The model under review builds one solid part; all positions refer to its coordinate system, in mm. A direction names the side the tool comes from. Round coordinates to 2 decimals unless told otherwise and drop trailing zeros. Loops run counter-clockwise (first coordinate to the right, second up) from the corner with the lowest first, then second, coordinate; pieces in that order, holes last. Notation, with made-up numbers: M 74.5,88.5 L 104.5,88.5 A20 ccw 104.5,96.5 Z; hole C 28,53 d3. An arc over 180 degrees is marked long. Return JSON: item names as keys, results as strings. Group by question number.
Q1. Consider section B-B (x = -6). State the section outline as (y, z) points.
Q2. Consider section A-A (z = -6). State the section outline as (x, y) points.
Q3. Consider section D-D (z = 10.5). State the section outline as (x, y) points, and give its area (3 significant figures).
Q4. To check wall thickness, follow line 1 along X through (y, z) = (1.5, -6); line 2 along X through (y, z) = (3.25, -15); line 3 along Z through (x, y) = (5, 1). State the ranges of each line that lie inside material, in increasing order.
Q5. Clearance check with flat-ended pins moving along their axes: pin 1 Ø1.8 at (y, z) = (3.5, 14.5) entering from +X; pin 2 Ø5.5 at (x, z) = (4, -6) entering from -Y; pin 3 Ø1 at (y, z) = (3.5, 3.5) entering from -X; pin 4 Ø5.5 at (x, z) = (-8, -7) entering from -Y. State where each tip first meets the part, or that it passes through.
Q6. Consider section C-C (y = 5). State the section outline as (x, z) points (3 decimals).
Q7. Draft analysis for pull direction Z (two halves, no side actions). For faces 5 (the face through (21, 3, 5)), 6 (the face through (4, 4, -4)), 7 (the face through (-9, 5, -21)), 8 (the face through (-13.12, 0.64, -18.03)), state which applies: pulls with the +Z half, pulls with the -Z half, needs draft (parallel to the pull), parting line crosses it, or undercut.
Q8. For faces 1 (the face through (-18, 1.3, -10)), 2 (the face through (-8.48, 4.99, 8.12)), 3 (the face through (6.828, 3, 14)), 4 (the face through (-3.97, 5.01, 1.79)), list the 3-axis set-ups (+Z, -Z, +X, -X, +Y, -Y) from which the entire face can be reached by the end or side of a thin tool; tool diameter is ignored.
from build123d import *

# Parameters (mm, degrees)
SKETCH2_W           = 44
SKETCH2_H           = 44
BOSS_EXTRUDE1_DEPTH = 6
CHAMFER1_SIZE       = 18
SKETCH3_R           = 8
CUT_EXTRUDE1_DEPTH  = 32.685959036
SKETCH4_R           = 9.1
CUT_EXTRUDE2_DEPTH  = 1.3
CUT_EXTRUDE3_DEPTH  = 32.685959036
SKETCH7_R           = 1.7
CUT_EXTRUDE4_DEPTH  = 32.685959036
SKETCH8_R           = 3
CUT_EXTRUDE5_DEPTH  = 2
CHAMFER2_SIZE       = 2


with BuildPart() as part:
    # Sketch2 → Boss-Extrude1 (new body)
    with BuildSketch(Plane(origin=(0, 0, 0), x_dir=(1, 0, 0), z_dir=(0, 1, 0))):
        Rectangle(SKETCH2_W, SKETCH2_H)
    extrude(amount=BOSS_EXTRUDE1_DEPTH)

    # Chamfer1
    chamfer1_edges = [part.edges().sort_by_distance(p)[0] for p in [
        (22, 3, 22),
    ]]
    chamfer(chamfer1_edges, length=CHAMFER1_SIZE)

    # Sketch3 → Cut-Extrude1 (cut, through all)
    with BuildSketch(Plane(origin=(0, 6, 0), x_dir=(1, 0, 0), z_dir=(0, 1, 0))):
        with Locations(Location((-9.629833996, 9.625, 0), (0, 0, 270))):
            Circle(SKETCH3_R)
    extrude(amount=-CUT_EXTRUDE1_DEPTH, mode=Mode.SUBTRACT)

    # Sketch4 → Cut-Extrude2 (cut)
    with BuildSketch(Plane(origin=(0, 0, 0), x_dir=(-1, 0, 0), z_dir=(0, -1, 0))):
        with Locations(Location((9.629833996, 9.625, 0), (0, 0, 90))):
            Circle(SKETCH4_R)
    extrude(amount=-CUT_EXTRUDE2_DEPTH, mode=Mode.SUBTRACT)

    # Sketch5 → Cut-Extrude3 (cut, through all)
    with BuildSketch(Plane(origin=(0, 6, 0), x_dir=(1, 0, 0), z_dir=(0, 1, 0))):
        Polygon((-14, 22), (-22, 14), (-22, 22), align=None)
    extrude(amount=-CUT_EXTRUDE3_DEPTH, mode=Mode.SUBTRACT)

    # Sketch7 → Cut-Extrude4 (cut, through all)
    with BuildSketch(Plane(origin=(0, 6, 0), x_dir=(1, 0, 0), z_dir=(0, 1, 0))):
        with Locations(Location((4, 6, 0), (0, 0, 270))):
            Circle(SKETCH7_R)
        with Locations(Location((-6, -4, 0), (0, 0, 270))):
            Circle(SKETCH7_R)
        Polygon((-4, 22), (22, -4), (22, 22), align=None)
        Polygon((-22, 4), (4, -22), (-22, -22), align=None)
        Polygon((19.171572875, -6.828427125), (9.656854249, -6.828427125), (6.828427125, -9.656854249), (6.828427125, -19.171572875), align=None)
    extrude(amount=-CUT_EXTRUDE4_DEPTH, mode=Mode.SUBTRACT)

    # Sketch8 → Cut-Extrude5 (cut)
    with BuildSketch(Plane(origin=(0, 6, 0), x_dir=(1, 0, 0), z_dir=(0, 1, 0))):
        with Locations(Location((4, 6, 0), (0, 0, 270))):
            Circle(SKETCH8_R)
        with Locations(Location((-6, -4, 0), (0, 0, 270))):
            Circle(SKETCH8_R)
    extrude(amount=-CUT_EXTRUDE5_DEPTH, mode=Mode.SUBTRACT)

    # Chamfer2
    chamfer2_edges = [part.edges().sort_by_distance(p)[0] for p in [
        (-22, 6, -9),
        (-18, 6, -18),
        (-9, 6, -22),
        (-9, 6, 9),
        (9, 6, -9),
    ]]
    chamfer(chamfer2_edges, length=CHAMFER2_SIZE)


solid = part.part
Values:
{
 "1": {"outline": "M 0,-22 L 4,-22 L 6,-20 L 6,-16.75 L 1.3,-16.75 L 1.3,-17.97 L 0,-17.97 Z; M 0,-1.28 L 1.3,-1.28 L 1.3,-2.5 L 6,-2.5 L 6,1 L 4,1 L 4,2.3 L 0,2.3 Z; M 0,5.7 L 4,5.7 L 4,7 L 6,7 L 6,9.17 L 4,12 L 0,12 Z"},
 "2": {"outline": "M -22,0 L -17.98,0 L -17.98,1.3 L -16.76,1.3 L -16.76,6 L -20,6 L -22,4 Z; M -2.5,1.3 L -1.28,1.3 L -1.28,0 L 2.3,0 L 2.3,4 L 1,4 L 1,6 L -2.5,6 Z; M 5.7,0 L 12,0 L 12,4 L 9.17,6 L 7,6 L 7,4 L 5.7,4 Z"},
 "3": {"outline": "M -7.5,0 L 6.83,0 L 6.83,6 L -4.67,6 L -7.5,4 Z", "area": "83.1 mm2"},
 "4": {"line 1": "x = -22 to -16.76, -2.5 to 2.3, 5.7 to 12", "line 2": "x = -21 to -15.56, -3.7 to 3", "line 3": "z = -13 to -7.37, -4.63 to 21"},
 "5": {"pin 1": "stops at x = 6.83", "pin 2": "stops at y = 0", "pin 3": "stops at x = -15", "pin 4": "passes through"},
 "6": {"outline": "M -21,-13.586 L -13.586,-21 L -4.414,-21 L 21.293,4.707 L 19.172,6.828 L 9.657,6.828 L 6.828,9.657 L 6.828,19.172 L 4.707,21.293 L -21,-4.414 Z; hole C -9.63,-9.625 d16; hole C -6,4 d6; hole C 4,-6 d6"},
 "7": {"face 5": "pulls with the +Z half", "face 6": "undercut", "face 7": "pulls with the -Z half", "face 8": "undercut"},
 "8": {"face 1": "-Y", "face 2": "+Z, -X, +Y", "face 3": "+Z, +X, +Y, -Y", "face 4": "+Y"}
}
